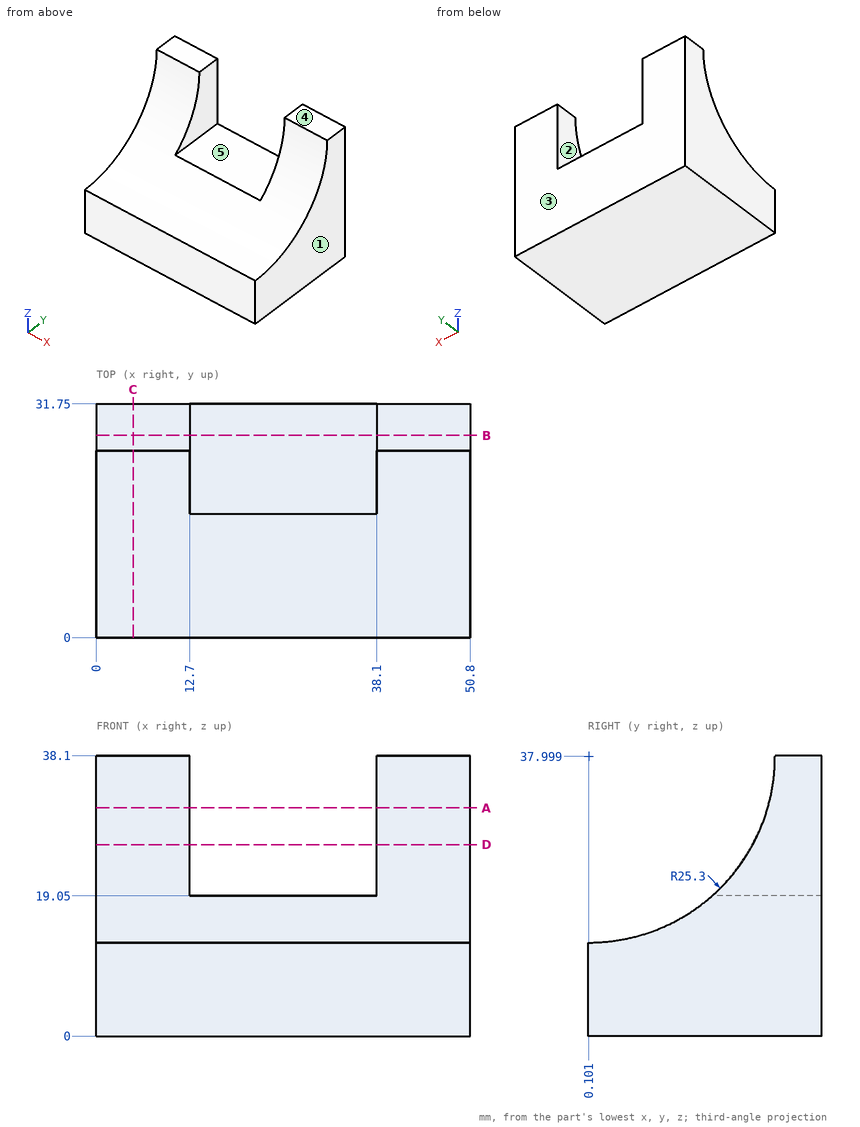
Design review of the part shown in the three views and the two pictorial views. Dimensions are in mm from the part's minimum x, y and z. A direction names the side the tool comes from. Round coordinates to 2 decimals unless told otherwise and drop trailing zeros. Write each loop counter-clockwise with the first axis right and the second up, starting at its lowest first coordinate (ties: lowest second). Pieces come first, ordered by that corner, then holes. Notation, with made-up numbers: (66.25, 58) - (74.25, 58) arc R18 ccw to (74.25, 89) - close; hole circle Ø11 at (61, -8.5). An arc over 180 degrees is marked (long way). Answer as CSV lines item,"result". Start each with the question number.
(1) Add section C-C, the plane x = 5. State the section outline as (y, z) points, plus the area to 3 significant figures.
(2) For line 1 (X direction, y = 28.5, z = 32.5); line 2 (Z direction, x = 32, y = 30); line 3 (Y direction, x = 41.5, z = 35.5), list the stretches that pass through material, from the lowest coordinate up.
(3) Machinability: for the marked faces 4 and 5, which of the approach directions +Z, -Z, +X, -X, +Y, -Y give a long, thin tool a straight path to every point of the face, cutting with its end or side? Answer none if there is none.
(4) Mouldability with a two-part tool opening along X and no side actions: class the marked faces 1, 2 and 3 as +X half, -X half, draft (parallel to the pull), parting line (faces both ways), or undercut.
(5) For pin 1 (3 mm diameter, centred on y = 22.5, z = 26.5, fed in from -X); pin 2 (10 mm diameter, centred on x = 16.5, z = 22, fed in from -Y); pin 3 (3 mm diameter, centred on x = 34.5, y = 19.5, fed in from +Z), all flat-tipped, find the tip position at first contact; note any pin that passes through.
(6) Add section D-D, the plane z = 26. State the section outline as (x, y) points.
(7) Add section A-A, the plane z = 31. State the section outline as (x, y) points.
(8) Add section B-B, the plane y = 27.5. State the section outline as (x, z) points.
From the geometry:
1,outline,"(0, 0) - (31.75, 0) - (31.75, 38.1) - (25.4, 38.1) arc R25.3 cw to (0, 12.7) - close"
1,area,"702 mm²"
2,line 1,"x = 0 to 12.7, 38.1 to 50.8"
2,line 2,"z = 0 to 19.05"
2,line 3,"y = 25.28 to 31.75"
3,face 4,"+Z, +X, -X, +Y, -Y"
3,face 5,"+Z, +Y, -Y"
4,face 1,"+X half"
4,face 2,"undercut"
4,face 3,"draft"
5,pin 1,"stops at x = 0"
5,pin 2,"stops at y = 14.21"
5,pin 3,"stops at z = 19.05"
6,outline,"(0, 22.37) - (12.7, 22.37) - (12.7, 31.75) - (0, 31.75) - close; (38.1, 22.37) - (50.8, 22.37) - (50.8, 31.75) - (38.1, 31.75) - close"
7,outline,"(0, 24.41) - (12.7, 24.41) - (12.7, 31.75) - (0, 31.75) - close; (38.1, 24.41) - (50.8, 24.41) - (50.8, 31.75) - (38.1, 31.75) - close"
8,outline,"(0, 0) - (50.8, 0) - (50.8, 38.1) - (38.1, 38.1) - (38.1, 19.05) - (12.7, 19.05) - (12.7, 38.1) - (0, 38.1) - close"
